Design review of the part built by this model. Coordinates are the model's own, in mm. Coordinates: 2 decimals unless noted, no trailing zeros. Loops run counter-clockwise (first coordinate to the right, second up) from the corner with the lowest first, then second, coordinate; pieces in that order, holes last. Notation, with made-up numbers: M -13.5,0.25 L 31.5,0.25 A20 cw 31.5,15.25 Z; hole C 33,-34.5 d7. An arc over 180 degrees is marked long. Answer as CSV lines item,"result". Start each with the question number.
from build123d import *

# Parameters (mm, degrees)
F0_W     = 350
F0_H     = 350
F1_DEPTH = 3
F2_W     = 260
F2_H     = 220
F3_DEPTH = 25
F5_D     = 3
F4_R     = 12.5
F6_DEPTH = 25


with BuildPart() as f1:
    # F0 (on Top) → F1 (new body)
    with BuildSketch(Plane.XY):
        Rectangle(F0_W, F0_H)
    extrude(amount=F1_DEPTH)

    # F2 (on face) → F3 (cut)
    with BuildSketch(Plane.XY.offset(3)):
        with Locations((0, -10)):
            Rectangle(F2_W, F2_H)
    extrude(amount=-F3_DEPTH, mode=Mode.SUBTRACT)

    # F5 (through all)
    with Locations(Plane.XY.offset(3)):
        with Locations((-161, 161), (-161, 130), (-130, 130), (-130, 161), (130, 161), (161, 161), (161, 130), (130, 130), (-15.5, 161), (-15.5, 130), (15.5, 130), (15.5, 161)):
            Hole(F5_D / 2)

    # F4 (on face) → F6 (cut)
    with BuildSketch(Plane.XY.offset(3)):
        with Locations((-145.5, 145.5)):
            Circle(F4_R)
        with Locations((145.5, 145.5)):
            Circle(F4_R)
        with Locations((0, 145.5)):
            Circle(F4_R)
    extrude(amount=-F6_DEPTH, mode=Mode.SUBTRACT)


solid = f1.part
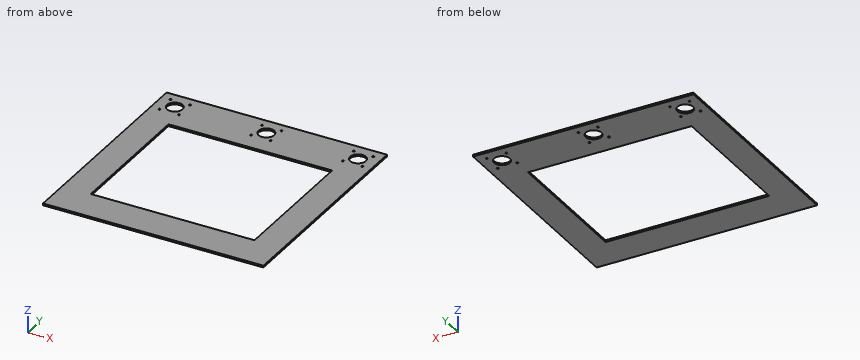
Item 1: Add section C-C (z = 1.2). Give the number of separate pieces and of enclosed holes in the cut face, plus the area to 3 significant figures.
Item 2: Add section B-B (x = 145.5). Give the boundary of the cut face in (y, z), plus the area to 3 significant figures.
Item 3: Add section D-D (y = 145.5). Give the boundary of the cut face in (x, z).
Item 4: Add section A-A (y = 93.5). Give the boundary of the cut face in (x, z).
Item 5: For pin 1 (2.5 mm diameter, centred on x = 161, y = 130, fed in from +Z); pin 2 (12 mm diameter, centred on x = 72.5, y = -126, fed in from -Z), all flat-tipped, find the tip position at first contact; note any pin that passes through.
Item 6: For line 1 along Y through (x, z) = (0, 2.45); line 2 along Y through (x, z) = (-161, 0.8); line 3 along X through (y, z) = (98.5, 1.3), list the stretches that pass through material, from the lowest coordinate up. Write a range as from..to.
Response:
1,separate pieces,"1"
1,enclosed holes,"16"
1,area,"63,700 mm²"
2,outline,"M -175,0 L 133,0 L 133,3 L -175,3 Z; M 158,0 L 175,0 L 175,3 L 158,3 Z"
2,area,"975 mm²"
3,outline,"M -175,0 L -158,0 L -158,3 L -175,3 Z; M -133,0 L -12.5,0 L -12.5,3 L -133,3 Z; M 12.5,0 L 133,0 L 133,3 L 12.5,3 Z; M 158,0 L 175,0 L 175,3 L 158,3 Z"
4,outline,"M -175,0 L -130,0 L -130,3 L -175,3 Z; M 130,0 L 175,0 L 175,3 L 130,3 Z"
5,pin 1,"through"
5,pin 2,"z = 0"
6,line 1,"-175..-120, 100..133, 158..175"
6,line 2,"-175..128.5, 131.5..159.5, 162.5..175"
6,line 3,"-175..-130, 130..175"
